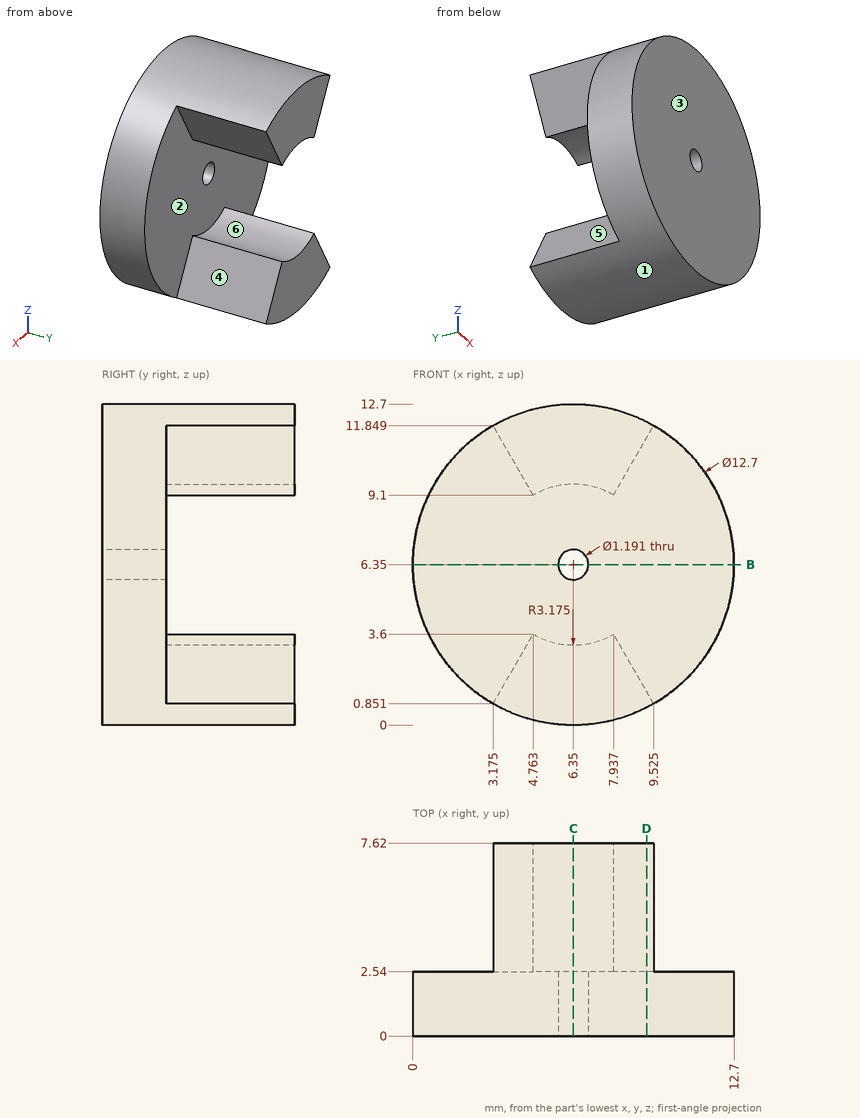
Geometry: see drawing. Coordinates: mm, zero at the bounding-box minimum. A direction names the side the tool comes from. Coordinates: 2 decimals unless noted, no trailing zeros. Loops run counter-clockwise (first coordinate to the right, second up) from the corner with the lowest first, then second, coordinate; pieces in that order, holes last. Notation, with made-up numbers: (2.25, 48.25) - (16.25, 48.25) arc R22 cw to (16.25, 54.25) - close; hole circle Ø8 at (87, -27.75). An arc over 180 degrees is marked (long way). Answer in a Markdown table with one row per item.
(1) Cut plane D-D on x = 9.25. Output: boundary loops of the cut face in (y, z).
Model answer:
| item | result |
|---|---|
| outline | (0, 0.7) - (7.62, 0.7) - (7.62, 1.33) - (2.54, 1.33) - (2.54, 11.37) - (7.62, 11.37) - (7.62, 12) - (0, 12) - close |
(2) Cut plane C-C on x = 6.35. Output: boundary loops of the cut face in (y, z) (1 decimal).
Model answer:
| item | result |
|---|---|
| outline | (0, 0) - (7.6, 0) - (7.6, 3.2) - (2.5, 3.2) - (2.5, 5.8) - (0, 5.8) - close; (0, 6.9) - (2.5, 6.9) - (2.5, 9.5) - (7.6, 9.5) - (7.6, 12.7) - (0, 12.7) - close |
(3) Mould query, pull axis Z, two halves, no side actions, for the marked faces 1, 2 and 3. Classes: pulls with the +Z half, pulls with the -Z half, needs draft (parallel to the pull), parting line crosses it, or undercut.
Model answer:
| item | result |
|---|---|
| face 1 | parting line crosses it |
| face 2 | undercut |
| face 3 | needs draft |
(4) Set-up query: the marked faces 4, 5 and 6. Return all of +Z, -Z, +X, -X, +Y, -Y with unobstructed straight access to the full face (end or side cutting, diameter ignored); none if empty.
Model answer:
| item | result |
|---|---|
| face 4 | +X, +Y |
| face 5 | -X, +Y |
| face 6 | +Y |
(5) Cut plane B-B on z = 6.35. Output: boundary loops of the cut face in (x, y) (1 decimal).
Model answer:
| item | result |
|---|---|
| outline | (0, 0) - (5.8, 0) - (5.8, 2.5) - (0, 2.5) - close; (6.9, 0) - (12.7, 0) - (12.7, 2.5) - (6.9, 2.5) - close |
(6) Pin query (flat end, axial travel): P1, Ø4, axis at x = 10, y = 5.5, coming from the +Z side; P2, Ø1, axis at y = 1, z = 2, coming from the +X side. Return the tip coordinate at first contact, or that it passes through.
Model answer:
| item | result |
|---|---|
| P1 | stops at z = 12.48 |
| P2 | stops at x = 11.4 |
(7) Material intervals for L1, parallel to X at y = 1.05, z = 6.35 (1 decimal); L2, parallel to Y at x = 8, z = 7, sorted ascending. Write a range as from..to.
Model answer:
| item | result |
|---|---|
| L1 | x = 0..5.8, 6.9..12.7 |
| L2 | y = 0..2.54 |
